Check sheet for the modelled part. Datum: model origin and axes. Units: mm. A direction names the side the tool comes from. Coordinates: 2 decimals unless noted, no trailing zeros. Write each loop counter-clockwise with the first axis right and the second up, starting at its lowest first coordinate (ties: lowest second). Pieces come first, ordered by that corner, then holes. Notation, with made-up numbers: M 37,50.5 L 54,50.5 A18 ccw 54,72.5 Z; hole C 36.5,63 d7. An arc over 180 degrees is marked long. Answer as CSV lines item,"result". Start each with the question number.
Q1. Sectioned sample at B-B, the plane x = 244. Record the cut outline in (y, z).
Q2. Sectioned sample at D-D, the plane x = 263.5. Record the cut outline in (y, z).
Q3. Depth check by flat-ended pin: pin 1 Ø4 at (x, y) = (257, 74) entering from -Z; pin 2 Ø1 at (y, z) = (79.5, 2.5) entering from -X. Enter the tip coordinate at first touch or a pass-through.
Q4. Thickness scan on line 1 along Y through (x, z) = (268.5, 0.8); line 2 along Y through (x, z) = (244.5, 2.4); line 3 along X through (y, z) = (73.5, 2.4). Record the ranges inside material, lowest first. Write a range as from..to.
Q5. Mould release check, pull along Y, two halves, no side actions. Record for faces 4 (the cylindrical face through (241.527, 82.649, 1.479)), 5 (the cylindrical face through (263.43, 80.35, 1.48)), 6 (the cylindrical face through (252.344, 79.811, 1.479)): pulls with the +Y half, pulls with the -Y half, needs draft (parallel to the pull), parting line crosses it, or undercut.
Q6. Access from +Z, -Z, +X, -X, +Y, -Y to the whole of each face (thin tool, end or side, straight path). Record for faces 1 (the flat face through (253.499, 82.564, 1.479)), 2 (the flat face through (251.786, 76.854, 1.479)), 3 (the flat face through (255.592, 79.627, 1.479)).
Q7. Sectioned sample at A-A, the plane y = 73.25. Record the cut outline in (x, z).
Q8. Sectioned sample at C-C, the plane z = 0.5. Record the cut outline in (x, y).
from build123d import *

# Parameters (mm, degrees)
SKETCH_1_R      = 3.6
SKETCH_1_R_2    = 1.25
EXTRUDE_1_DEPTH = 3


with BuildPart() as part:
    # 草圖1 → 填料-伸長1 (new body)
    with BuildSketch(Plane.XY):
        with BuildLine():
            Line((243.635524691, 78.984013539), (260.167543031, 74.664105375))
            ThreePointArc((260.167543031, 74.664105375), (261.762807038, 73.939164867), (263.0099811, 72.708326596))
            ThreePointArc((263.0099811, 72.708326596), (264.804382383, 71.148673452), (267.027735224, 70.306595047))
            ThreePointArc((267.027735224, 70.306595047), (267.669348827, 70.295848059), (268.307919069, 70.359184927))
            ThreePointArc((268.307919069, 70.359184927), (271.821757968, 72.430801884), (272.972563608, 76.344151728))
            ThreePointArc((272.972563608, 76.344151728), (271.674549014, 79.439761285), (268.83007541, 81.222066065))
            ThreePointArc((268.83007541, 81.222066065), (266.927260325, 81.319865813), (265.086550743, 80.827871636))
            ThreePointArc((265.086550743, 80.827871636), (263.401602385, 80.346994525), (261.654207062, 80.477007409))
            Line((261.654207062, 80.477007409), (245.112048777, 84.71112347))
            ThreePointArc((245.112048777, 84.71112347), (241.510232103, 82.585830461), (243.635524691, 78.984013539))
        make_face()
        with Locations((267.499543018, 75.885430609)):
            Circle(SKETCH_1_R, mode=Mode.SUBTRACT)
        with Locations((244.373787095, 81.847568395)):
            Circle(SKETCH_1_R_2, mode=Mode.SUBTRACT)
        with BuildLine():
            Line((257.981059369, 79.010683825), (253.134508891, 80.260187472))
            ThreePointArc((253.134508891, 80.260187472), (252.340612803, 79.796798865), (252.80400141, 79.002902777))
            Line((252.80400141, 79.002902777), (257.650550117, 77.753399602))
            ThreePointArc((257.650550117, 77.753399602), (258.444446854, 78.216787087), (257.981059369, 79.010683825))
        make_face(mode=Mode.SUBTRACT)
    extrude(amount=EXTRUDE_1_DEPTH)


solid = part.part
Output:
1,outline,"M 78.89,0 L 80.65,0 L 80.65,3 L 78.89,3 Z; M 83.04,0 L 84.78,0 L 84.78,3 L 83.04,3 Z"
2,outline,"M 72.16,0 L 80.36,0 L 80.36,3 L 72.16,3 Z"
3,pin 1,"stops at z = 0"
3,pin 2,"stops at x = 242.06"
4,line 1,"y = 70.39..72.43, 79.34..81.28"
4,line 2,"y = 78.76..80.6, 83.09..84.8"
4,line 3,"x = 262.31..264.8, 270.2..272.48"
5,face 4,"parting line crosses it"
5,face 5,"pulls with the +Y half"
5,face 6,"undercut"
6,face 1,"+Z, -Z, +Y"
6,face 2,"+Z, -Z, -X, -Y"
6,face 3,"+Z, -Z"
7,outline,"M 262.57,0 L 265.05,0 L 265.05,3 L 262.57,3 Z; M 269.95,0 L 272.35,0 L 272.35,3 L 269.95,3 Z"
8,outline,"M 243.64,78.98 L 260.17,74.66 A5 cw 263.01,72.71 A6.76 ccw 267.03,70.31 A5.55 ccw 268.83,81.22 A6.12 ccw 265.09,80.83 A5 cw 261.65,80.48 L 245.11,84.71 A2.96 ccw Z; hole C 244.37,81.85 d2.5; hole M 252.8,79 L 257.65,77.75 A0.65 ccw 257.98,79.01 L 253.13,80.26 A0.65 ccw Z; hole C 267.5,75.89 d7.2"
